from build123d import *

# Parameters (mm, degrees)
SKETCH2_R           = 14.5
BOSS_EXTRUDE1_DEPTH = 29
SKETCH5_R           = 4
BOSS_EXTRUDE2_DEPTH = 5
FILLET1_R           = 1
SKETCH8_R           = 7
CUT_EXTRUDE1_DEPTH  = 25


with BuildPart() as part:
    # Sketch2 → Boss-Extrude1 (new body)
    with BuildSketch(Plane.XY):
        with Locations(Location((0, 0, 0), (0, 0, 180))):
            Circle(SKETCH2_R)
    extrude(amount=BOSS_EXTRUDE1_DEPTH)

    # Sketch5 → Boss-Extrude2 (add)
    with BuildSketch(Plane.XY):
        with BuildLine():
            Line((0, 14.5), (0, -14.5))
            Line((0, -14.5), (-38.508744426, -10.953649377))
            ThreePointArc((-38.508744426, -10.953649377), (-48.5, 0), (-38.508744426, 10.953649377))
            Line((-38.508744426, 10.953649377), (0, 14.5))
        make_face()
        with Locations((-43.5, 0)):
            Circle(SKETCH5_R, mode=Mode.SUBTRACT)
    extrude(amount=BOSS_EXTRUDE2_DEPTH)

    # Fillet1
    fillet1_edges = [part.edges().sort_by_distance(p)[0] for p in [
        (-11.15009107, -9.269599189, 5),
    ]]
    fillet(fillet1_edges, radius=FILLET1_R)

    # Sketch8 → Cut-Extrude1 (cut)
    with BuildSketch(Plane.XY.offset(29)):
        Circle(SKETCH8_R)
    extrude(amount=-CUT_EXTRUDE1_DEPTH, mode=Mode.SUBTRACT)


solid = part.part
Read the model definition and answer for the solid it produces. Units are mm, in the model's axes. A direction names the side the tool comes from. Round coordinates to 2 decimals unless told otherwise and drop trailing zeros. Order: outer loops, then holes, each group sorted by start corner. A loop starts at its lowest first (then second) coordinate and runs counter-clockwise, first axis right, second up.
1) For faces 4 (the face through (-48.5, -0.2, 2.5)), 5 (the face through (14.486, -0.638, 14.297)), determine the directions among +Z, -Z, +X, -X, +Y, -Y from which every point of the face is accessible in a straight line to the end or side of a thin tool.
2) Straight lines are drawn through the part: L1, parallel to Y at x = 0, z = 23.5; L2, parallel to Z at x = -27, y = 0.75; L3, parallel to Y at x = -3, z = 5. For each, find the intervals that lie inside material, in ascending order.
3) The mould has two halves that part along Y. Classify faces 1 (the face through (-3, -7, 29)), 2 (the face through (6.466, -2.681, 16.675)), 3 (the face through (-20.327, -12.628, 2.291)): released by +Y, released by -Y, zero draft, split by the parting line, or undercut.
4) The part is cut by section C-C on z = 10. Write down the section's boundary in (x, y).
5) The part is cut by section A-A on y = 0. Write down the section's boundary in (x, z), plus the area to 3 significant figures.
6) Flat-ended cylindrical pins translate along their axes: pin 1 (8.5 mm diameter, centred on x = -37, y = 2, fed in from +Z); pin 2 (1.5 mm diameter, centred on y = 11, z = 6.5, fed in from -X); pin 3 (2 mm diameter, centred on y = 7, z = 6.5, fed in from +X). Find the tip coordinate at first contact, or state that the pin passes through.
7) The part is cut by section B-B on x = 0. Write down the section's boundary in (y, z).
8) The part is cut by section D-D on x = -43.5. Write down the section's boundary in (y, z).
Resolved:
1. face 4: +Z, -Z, -X
1. face 5: +Z
2. L1: y = -14.5 to -7, 7 to 14.5
2. L2: z = 0 to 5
2. L3: y = -14.22 to -6.32, 6.32 to 14.22
3. face 1: zero draft
3. face 2: undercut
3. face 3: released by -Y
4. outline: circle Ø29 at (0, 0); hole circle Ø14 at (0, 0)
5. outline: (-48.5, 0) - (-47.5, 0) - (-47.5, 5) - (-48.5, 5) - close; (-39.5, 0) - (14.5, 0) - (14.5, 29) - (7, 29) - (7, 4) - (-7, 4) - (-7, 29) - (-14.5, 29) - (-14.5, 6) arc R1 cw to (-15.5, 5) - (-39.5, 5) - close
5. area: 621 mm2
6. pin 1: stops at z = 5
6. pin 2: stops at x = -10.26
6. pin 3: stops at x = 13.2
7. outline: (-14.5, 0) - (14.5, 0) - (14.5, 29) - (7, 29) - (7, 4) - (-7, 4) - (-7, 29) - (-14.5, 29) - close
8. outline: (-9.22, 0) - (-4, 0) - (-4, 5) - (-9.22, 5) - close; (4, 0) - (9.22, 0) - (9.22, 5) - (4, 5) - close
